```python
from build123d import *

# Parameters (mm, degrees)
SKETCH_1_W          = 260
SKETCH_1_H          = 40
EXTRUDE_1_DEPTH     = 2
SKETCH_3_R          = 2
CUT_EXTRUDE_2_DEPTH = 2
CUT_EXTRUDE_3_DEPTH = 132.544669219
FILLET_1_R          = 3


with BuildPart() as part:
    # 草图1 → 凸台-拉伸1 (new body)
    with BuildSketch(Plane.XY):
        Rectangle(SKETCH_1_W, SKETCH_1_H)
    extrude(amount=EXTRUDE_1_DEPTH)

    # 草图3 → 切除-拉伸2 (cut)
    with BuildSketch(Plane.XY.offset(2)):
        with Locations((-122.5, 14)):
            Circle(SKETCH_3_R)
        with Locations((-122.5, -16)):
            Circle(SKETCH_3_R)
        with Locations(Location((122.5, -16, 0), (0, 0, 180))):
            Circle(SKETCH_3_R)
        with Locations(Location((122.5, 14, 0), (0, 0, 180))):
            Circle(SKETCH_3_R)
    extrude(amount=-CUT_EXTRUDE_2_DEPTH, mode=Mode.SUBTRACT)

    # 草图4 → 切除-拉伸3 (cut, through all)
    with BuildSketch(Plane.XY.offset(2)):
        with BuildLine():
            Line((-80, 7.5), (80, 7.5))
            ThreePointArc((80, 7.5), (87.5, 0), (80, -7.5))
            Line((80, -7.5), (-80, -7.5))
            ThreePointArc((-80, -7.5), (-87.5, 0), (-80, 7.5))
        make_face()
    extrude(amount=-CUT_EXTRUDE_3_DEPTH, mode=Mode.SUBTRACT)

    # 圆角1
    fillet_1_edges = [part.edges().sort_by_distance(p)[0] for p in [
        (130, -20, 1),
        (-130, -20, 1),
        (-130, 20, 1),
        (130, 20, 1),
    ]]
    fillet(fillet_1_edges, radius=FILLET_1_R)


solid = part.part
```
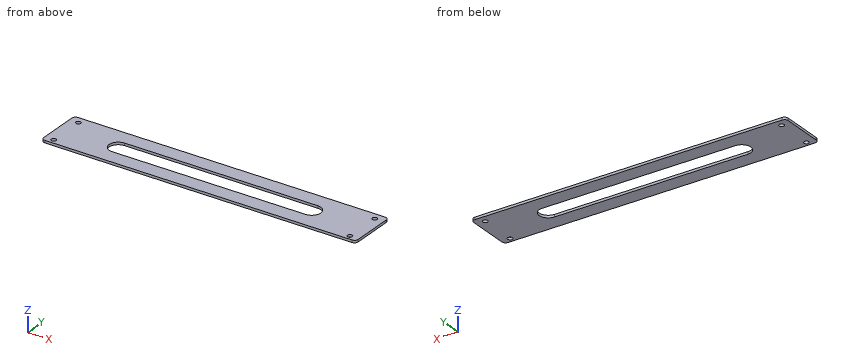
Build history of the part. All positions in model axes, mm. Give positions to 0.01 mm unless a question says otherwise; leave off trailing zeros. Loops run counter-clockwise (first coordinate to the right, second up) from the corner with the lowest first, then second, coordinate; pieces in that order, holes last. Notation, with made-up numbers: (11, 15) -> (20, 15) arc R12 cw to (20, 21) -> close; hole circle Ø4 at (-36, -7.75). An arc over 180 degrees is marked (long way). One line per question, with ' | ' between items. Start each with the question number.
1) Probe L1, parallel to Y at x = -122.5, z = 1; L2, parallel to Y at x = 21, z = 1.4; L3, parallel to X at y = -17, z = 0.6. List the from-to ranges inside material, lowest first.
2) Cut at C-C (z = 1.4). Give the cut face in (x, y).
3) Cut at A-A (x = -37.5). Give the cut face in (y, z), plus the area to 3 significant figures.
4) Pin check, flat tip, straight feed: pin 1 (6.5 mm diameter, centred on x = -122.5, y = -16, fed in from +Z). Stop position of the tip, or through.
5) Cut at B-B (y = 0). Give the cut face in (x, z), plus the area to 3 significant figures.
Return value:
1) L1: -20 to -18, -14 to 12, 16 to 20 | L2: -20 to -7.5, 7.5 to 20 | L3: -130 to -124.23, -120.77 to 120.77, 124.23 to 130
2) outline: (-130, -17) arc R3 ccw to (-127, -20) -> (127, -20) arc R3 ccw to (130, -17) -> (130, 17) arc R3 ccw to (127, 20) -> (-127, 20) arc R3 ccw to (-130, 17) -> close; hole circle Ø4 at (-122.5, -16); hole circle Ø4 at (-122.5, 14); hole (-80, -7.5) -> (80, -7.5) arc R7.5 ccw to (80, 7.5) -> (-80, 7.5) arc R7.5 ccw to start; hole circle Ø4 at (122.5, -16); hole circle Ø4 at (122.5, 14)
3) outline: (-20, 0) -> (-7.5, 0) -> (-7.5, 2) -> (-20, 2) -> close; (7.5, 0) -> (20, 0) -> (20, 2) -> (7.5, 2) -> close | area: 50.0 mm^2
4) pin 1: z = 2
5) outline: (-130, 0) -> (-87.5, 0) -> (-87.5, 2) -> (-130, 2) -> close; (87.5, 0) -> (130, 0) -> (130, 2) -> (87.5, 2) -> close | area: 170 mm^2
